The listing builds one solid part. Answer for the finished solid, in the listing's coordinates (mm). Give positions to 0.01 mm unless a question says otherwise; leave off trailing zeros. Order: outer loops, then holes, each group sorted by start corner. A loop starts at its lowest first (then second) coordinate and runs counter-clockwise, first axis right, second up. Notation, with made-up numbers: (-32, -30.75) - (-13, -30.75) arc R16 ccw to (-13, -23.75) - close; hole circle Ø8 at (9, 71.25). An arc over 180 degrees is marked (long way). Answer as CSV lines item,"result". Start each with the question number.
1. Section B-B on x = 0 is taken. Give the vertices of the cut face in (y, z).
2. Section D-D on z = -1.75 is taken. Give the vertices of the cut face in (x, y).
3. Consider line 1 along Y through (x, z) = (0.25, -7); line 2 along X through (y, z) = (19, -3); line 3 along Y through (x, z) = (-2.25, -4). Determine where each line is inside the solid, lowest interval first. Write a range as [from, to].
4. Flat-ended cylindrical pins translate along their axes: pin 1 (1 mm diameter, centred on x = 2.5, z = -1, fed in from -Y); pin 2 (4 mm diameter, centred on x = -2.5, y = 20.5, fed in from -Z); pin 3 (1.5 mm diameter, centred on x = -2, z = -1, fed in from -Y); pin 4 (1 mm diameter, centred on y = 22.5, z = -4.5, fed in from +X). Find the tip coordinate at first contact, or state that the pin passes through.
5. Section A-A on y = 21.5 is taken. Give the vertices of the cut face in (x, z).
6. Section C-C on z = -5.5 is taken. Give the vertices of the cut face in (x, y).
from build123d import *

# Parameters (mm, degrees)
SKETCH1_R           = 3.8
BOSS_EXTRUDE1_DEPTH = 3
SKETCH2_R           = 3.4
BOSS_EXTRUDE2_DEPTH = 5
FILLET1_R           = 1
CHAMFER1_SIZE       = 0.5


with BuildPart() as part:
    # Sketch1 → Boss-Extrude1 (new body)
    with BuildSketch(Plane.XY):
        with Locations((0, 21.5)):
            Circle(SKETCH1_R)
    extrude(amount=-BOSS_EXTRUDE1_DEPTH)

    # Sketch2 → Boss-Extrude2 (add)
    with BuildSketch(Plane(origin=(0, 0, -3), x_dir=(-1, 0, 0), z_dir=(0, 0, -1))):
        with Locations((0, 21.5)):
            Circle(SKETCH2_R)
    extrude(amount=BOSS_EXTRUDE2_DEPTH)

    # Fillet1
    fillet1_edges = [part.edges().sort_by_distance(p)[0] for p in [
        (3.4, 21.5, -8),
    ]]
    fillet(fillet1_edges, radius=FILLET1_R)

    # Chamfer1
    # the kernel refuses this chamfer: 0.5 mm, written as the material it takes off along each edge
    with BuildSketch(Plane(origin=(0, 21.5, -3), x_dir=(1, 0, 0), z_dir=(0, -1, 0))) as chamfer1_piece_1_section:
        Polygon((3.8 - CHAMFER1_SIZE, 0), (3.8, CHAMFER1_SIZE), (3.8, 0), align=None)
    chamfer1_piece_1 = revolve(axis=Axis((0, 21.5, -3), (0, 0, 1)), mode=Mode.PRIVATE)
    chamfer1_piece_1 = chamfer1_piece_1 - Plane(origin=(0, 21.5, -2.703116332), x_dir=(-1, 0, 0), z_dir=(0, 0, 1)) * Cylinder(3.4, 16, mode=Mode.PRIVATE)
    add(chamfer1_piece_1, mode=Mode.SUBTRACT)


solid = part.part
Checks:
1,outline,"(17.7, -2.5) - (18.1, -2.9) - (18.1, -7) arc R1 ccw to (19.1, -8) - (23.9, -8) arc R1 ccw to (24.9, -7) - (24.9, -2.9) - (25.3, -2.5) - (25.3, 0) - (17.7, 0) - close"
2,outline,"circle Ø7.6 at (0, 21.5)"
3,line 1,"y = [18.11, 24.89]"
3,line 2,"x = [-2.3, 2.3]"
3,line 3,"y = [18.95, 24.05]"
4,pin 1,"stops at y = 18.27"
4,pin 2,"stops at z = -8"
4,pin 3,"stops at y = 17.91"
4,pin 4,"stops at x = 3.36"
5,outline,"(-3.8, -2.5) - (-3.4, -2.9) - (-3.4, -7) arc R1 ccw to (-2.4, -8) - (2.4, -8) arc R1 ccw to (3.4, -7) - (3.4, -2.9) - (3.8, -2.5) - (3.8, 0) - (-3.8, 0) - close"
6,outline,"circle Ø6.8 at (0, 21.5)"
